Source: CAD feature listing. Evaluate the final solid. Frame: model axes, mm. Face numbers are marked on the shaded views. A direction names the side the tool comes from. Coordinates: 2 decimals unless noted, no trailing zeros. Write each loop counter-clockwise with the first axis right and the second up, starting at its lowest first coordinate (ties: lowest second). Pieces come first, ordered by that corner, then holes. Notation, with made-up numbers: (22, 18) - (37, 18) arc R24 ccw to (37, 30) - close; hole circle Ø10 at (56, 60.25). An arc over 180 degrees is marked (long way). One line per question, with ' | ' between items.
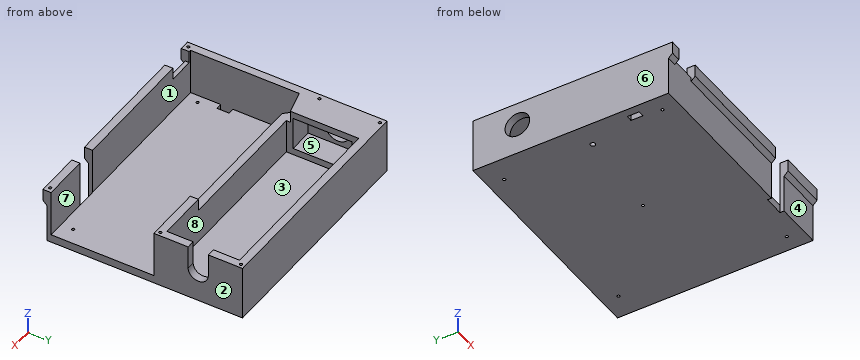
Autodesk Inventor part; units mm, degrees
ref_plane "YZ Plane" through (0, 0, 0) normal (1, 0, 0) x (0, 1, 0)
ref_plane "XZ Plane" through (0, 0, 0) normal (0, 1, 0) x (-1, 0, 0)
ref_plane "XY Plane" through (0, 0, 0) normal (0, 0, 1) x (1, 0, 0)
sketch "Skizze1" plane through (0, 0, 0) normal (0, 0, 1) x (1, 0, 0)
  line L0 (0, 0) -> (115, 0)
  line L1 (115, 0) -> (115, -97)
  line L2 (115, -97) -> (0, -97)
  line L3 (0, -97) -> (0, 0)
  dimension "d0" = 115
  dimension "d1" = 97
extrude "Extrusion1" add sketch "Skizze1" along normal blind 4
sketch "Skizze2" plane through (0, 0, 4) normal (0, 0, 1) x (1, 0, 0)
  line L0 (0, -97) -> (115, -97)
  line L1 (115, -97) -> (115, 0)
  line L2 (115, 0) -> (0, 0)
  line L3 (0, 0) -> (0, -97)
  line L4 (4, -44) -> (4, -95)
  line L5 (4, -95) -> (115, -95)
  line L6 (115, -97) -> (115, 0)
  line L7 (4, -44) -> (115, -44)
  line L8 (4, -40) -> (16, -40) construction
  line L9 (4, -40) -> (4, -36.6) construction
  line L10 (4, -4) -> (16, -4) construction
  line L11 (4, -7.4) -> (16, -7.4)
  line L12 (16, -7.4) -> (16, -4)
  line L13 (4, -36.6) -> (16, -36.6)
  line L14 (16, -36.6) -> (16, -40)
  line L15 (4, -36.6) -> (4, -7.4)
  line L16 (16, -40) -> (111, -40)
  line L17 (4, -7.4) -> (4, -4) construction
  line L18 (16, -4) -> (111, -4)
  line L19 (111, -4) -> (111, -40)
  point P0 (109.25, 0)
  point P1 (109.25, -40)
  dimension "d4" = 4
  dimension "d5" = 2
  dimension "d6" = 51
  dimension "d7" = 4
  dimension "d8" = 36
  dimension "d9" = 4
  dimension "d10" = 29.2
  dimension "d11" = 12
  dimension "d30" = 4
extrude "Extrusion2" add sketch "Skizze2" along normal blind 23 contours L3 L2 L1 L7 L4 L5 L0
sketch "Skizze4" plane through (0, 0, 4) normal (0, 0, 1) x (1, 0, 0)
  line L0 (4, -36.6) -> (16, -36.6)
  line L1 (4, -36.6) -> (16, -36.6)
  line L2 (16, -36.6) -> (16, -7.4)
  line L3 (16, -7.4) -> (4, -7.4)
  line L4 (4, -7.4) -> (4, -36.6)
  point P0 (0, 0)
  point P1 (16, -7.4)
extrude "Extrusion4" add sketch "Skizze4" along normal blind 3.3
sketch "Skizze5" plane through (4, -36.6, 27) normal (1, 0, 0) x (0, 0, -1)
  line L0 (0, 0) -> (0, 29.2)
  line L1 (0, 29.2) -> (3.3, 29.2)
  line L2 (3.3, 29.2) -> (3.3, 0)
  line L3 (3.3, 0) -> (0, 0)
  line L4 (0, 0) -> (0, 29.2)
  line L5 (19.7, 0) -> (0, 0)
  line L6 (19.7, 0) -> (19.7, 29.2)
  circle A0 centre (11.5, 14.6) radius 6.1
  line L7 (7.2229, 14.6) -> (16.7001, 14.6)
  line L8 (11.5, 24.1317) -> (11.5, 8.2548) construction
  point P0 (27, 36.6)
  dimension "d20" = 16.4
  dimension "d21" = 29.2
  dimension "d22" = 12.2
extrude "Extrusion5" cut sketch "Skizze5" against normal through all contours A0
extrude "Extrusion6" add sketch "Skizze5" along normal up to surface (12 mm away) contours L0 L1 L2 L3
sketch "Skizze6" plane through (0, 0, 27) normal (0, 0, 1) x (1, 0, 0)
  line L0 (4, -44) -> (115, -44)
  line L1 (111, -40) -> (16, -40)
  line L2 (86, -44) -> (16, -44)
  line L3 (16, -44) -> (16, -40)
  line L4 (16, -40) -> (86, -40)
  line L5 (86, -40) -> (86, -44)
  line L6 (4, -44) -> (4, -95)
  line L7 (0, -97) -> (115, -97)
  line L8 (14, -97) -> (7, -97)
  line L9 (115, -95) -> (4, -95)
  line L10 (92, -95) -> (82, -95)
  line L11 (82, -95) -> (82, -97)
  line L12 (82, -97) -> (92, -97)
  line L13 (92, -97) -> (92, -95)
  line L14 (115, -97) -> (115, -95)
  line L15 (5, -95) -> (18, -95)
  line L16 (18, -95) -> (18, -97)
  line L17 (18, -97) -> (5, -97)
  line L18 (5, -97) -> (5, -95)
  line L19 (0, 0) -> (0, -97)
  point P0 (109.25, -40)
  point P1 (86, -42)
  point P2 (86, -40)
  point P3 (82, -95)
  point P4 (5, -96)
  point P5 (18, -96)
  point P6 (5, -97)
  point P7 (18, -97)
  dimension "d27" = 70
  dimension "d41" = 10
  dimension "d42" = 23
  dimension "d65" = 13
  dimension "d66" = 5
extrude "Extrusion7" cut sketch "Skizze6" against normal blind 6 contours L3 L1 L5 L0
sketch "Skizze7" plane through (115, -97, 0) normal (1, 0, 0) x (0, 0, -1)
  arc A0 (-15.5, 80) -> (-15.5, 70) centre (-15.5, 75) ccw construction
  circle A1 centre (-15.5, 75) radius 6.1 construction
  line L0 (-15.5, 80) -> (-27, 80)
  line L1 (-27, 53) -> (-27, 97)
  line L2 (-15.5, 70) -> (-27, 70)
  arc A2 (-15.5, 70) -> (-15.5, 80) centre (-15.5, 75) ccw
  point P0 (0, 97)
  dimension "d31" = 10
extrude "Extrusion8" cut sketch "Skizze7" against normal blind 4
sketch "Skizze8" plane through (0, 0, 0) normal (0, 0, -1) x (-1, 0, 0)
  line L0 (0, -97) -> (-115, -97)
  line L1 (0, 0) -> (0, -97)
  line L2 (-115, 0) -> (0, 0)
  line L3 (-115, -97) -> (-115, 0)
  line L4 (-8, -8) -> (-8, -89) construction
  line L5 (-8, -89) -> (-107, -89) construction
  line L6 (-107, -89) -> (-107, -8) construction
  line L7 (-107, -8) -> (-8, -8) construction
  circle A0 centre (-107, -89) radius 0.7
  circle A1 centre (-8, -89) radius 0.7
  circle A2 centre (-103, -8) radius 0.7
  circle A3 centre (-12, -8) radius 0.7
  line L8 (-107, -8) -> (-8, -89) construction
  line L9 (-107, -89) -> (-8, -8) construction
  circle A4 centre (-57.5, -48.5) radius 0.7
  dimension "d34" = 8
  dimension "d35" = 1.4
  dimension "d36" = 4
  dimension "d37" = 4
extrude "Extrusion9" cut sketch "Skizze8" against normal blind 4 contours A0 | A1 | A2 | A3 | A4
extrude "Extrusion10" cut sketch "Skizze6" against normal blind 6 contours L9 L16 L7 L18
sketch "Skizze9" plane through (0, 0, 27) normal (0, 0, 1) x (1, 0, 0)
  line L0 (4, -95) -> (4, -44)
  line L1 (4, -44) -> (16, -44)
  line L2 (16, -44) -> (16, -4)
  line L3 (16, -4) -> (111, -4)
  line L4 (111, -4) -> (111, -17)
  line L5 (111, -40) -> (86, -40)
  line L6 (86, -40) -> (86, -44)
  line L7 (86, -44) -> (115, -44)
  line L8 (115, -44) -> (115, -27)
  line L9 (115, 0) -> (0, 0)
  line L10 (0, 0) -> (0, -97)
  line L11 (0, -97) -> (5, -97)
  line L12 (2.5, -2) -> (113, -2) construction
  line L13 (113, -2) -> (113, -97.1903) construction
  line L14 (113, -97.1903) -> (2.5, -97.1903) construction
  line L15 (2.5, -97.1903) -> (2.5, -2) construction
  circle A0 centre (2.5, -2) radius 0.7
  circle A1 centre (113, -2) radius 0.7
  circle A2 centre (113, -42) radius 0.7
  line L16 (113, -42) -> (2.5, -42) construction
  line L17 (4, -44) -> (16, -44) construction
  circle A3 centre (2.5, -32) radius 0.7
  line L18 (115, -27) -> (111, -27)
  line L19 (111, -27) -> (111, -40)
  line L20 (111, -17) -> (115, -17)
  line L21 (115, -17) -> (115, 0)
  line L22 (115, -97) -> (115, -95)
  line L23 (115, -95) -> (18, -95)
  line L24 (5, -97) -> (5, -95)
  line L25 (5, -95) -> (4, -95)
  line L26 (18, -95) -> (18, -97)
  line L27 (18, -97) -> (115, -97)
  dimension "d45" = 2
  dimension "d46" = 2.5
  dimension "d47" = 2
  dimension "d48" = 1.4
  dimension "d49" = 2
  dimension "d59" = 30
extrude "Extrusion11" cut sketch "Skizze9" against normal blind 4 contours A0 | A1 | A2 | A3
extrude "Extrusion12" cut sketch "Skizze6" against normal through all contours L9 L13 L7 L11
sketch "Skizze12" plane through (0, -97, 0) normal (0, -1, 0) x (1, 0, 0)
  line L0 (115, 4) -> (115, 27)
  line L1 (115, 27) -> (92, 27)
  line L2 (92, 27) -> (92, 21)
  line L3 (92, 21) -> (115, 21)
  line L4 (115, 21) -> (115, 27)
  line L5 (82, 0) -> (82, 27)
  line L6 (18, 27) -> (18, 21)
  line L7 (82, 27) -> (18, 27)
  line L8 (18, 27) -> (18, 21)
  line L9 (18, 21) -> (82, 21)
  line L10 (82, 21) -> (82, 27)
  line L11 (5, 21) -> (5, 27)
  line L12 (0, 0) -> (0, 27)
  line L13 (5, 21) -> (0, 21)
  line L14 (0, 21) -> (0, 27)
  line L15 (0, 27) -> (5, 27)
  line L16 (5, 27) -> (5, 21)
  point P0 (5, 27)
  point P1 (0, 21)
  dimension "d67" = 6
extrude "Extrusion15" add sketch "Skizze12" along normal blind 2
sketch "Skizze10" plane through (0, 0, 27) normal (0, 0, 1) x (1, 0, 0)
  line L0 (16, -44) -> (16, -4)
  line L1 (4, -44) -> (16, -44)
  line L2 (4, -95) -> (4, -44)
  line L3 (4, -44) -> (4, -41)
  line L4 (4, -41) -> (16, -38)
  point P0 (0, 0)
  dimension "d56" = 6
  dimension "d77" = 3
extrude "Extrusion13" cut sketch "Skizze10" against normal blind 6
sketch "Skizze11" plane through (0, 0, 4) normal (0, 0, 1) x (1, 0, 0)
  circle A0 centre (12, -52) radius 1.2
  line L0 (4, -44) -> (4, -95)
  line L1 (115, -44) -> (4, -44)
  point P0 (0, 0)
  dimension "d60" = 8
  dimension "d61" = 8
  dimension "d62" = 2.4
extrude "Extrusion14" cut sketch "Skizze11" against normal blind 4
sketch "Skizze13" plane through (0, 0, 27) normal (0, 0, 1) x (1, 0, 0)
  line L0 (5, -97) -> (0, -97)
  circle A0 centre (2.5, -97) radius 0.7
  circle A1 centre (2.5, -32) radius 0.7
  line L1 (0, 0) -> (0, -99)
  line L2 (115, -97) -> (92, -97)
  circle A2 centre (112.5, -97) radius 0.7
  line L3 (115, -95) -> (115, -99)
  dimension "d70" = 2.5
  dimension "d71" = 2.5
extrude "Extrusion16" cut sketch "Skizze13" against normal blind 5 contours A0 L0 | L0 A0 | A2 L2 | L2 A2
chamfer "Fasen1" distance 2 angle 45 3 edges at (2.5, -97, 21) (50, -97, 21) (103.5, -97, 21)
sketch "Skizze14" plane through (0, 0, 4) normal (0, 0, 1) x (1, 0, 0)
  line L0 (115, -44) -> (4, -44)
  line L1 (4, -74) -> (7, -74)
  line L2 (7, -74) -> (7, -80)
  line L3 (7, -80) -> (4, -80)
  line L4 (4, -80) -> (4, -44)
  line L5 (4, -95) -> (82, -95)
  point P0 (0, 0)
  point P1 (7, -44)
  point P2 (4, -74)
  dimension "d78" = 6
  dimension "d79" = 3
  dimension "d82" = 15
extrude "Extrusion17" cut sketch "Skizze14" against normal blind 10
sketch "Skizze16" plane through (0, 0, 21) normal (0, 0, 1) x (1, 0, 0)
  line L0 (86, -44) -> (4, -44)
  line L1 (4, -44) -> (4, -41)
  line L2 (4, -44) -> (4, -41)
  line L3 (4, -41) -> (9, -39.75)
  line L4 (4, -41) -> (16, -38)
  line L5 (9, -44.0784) -> (9, -39.75)
  point P0 (0, 0)
  point P1 (9, -41.9142)
  point P2 (9, -44)
  dimension "d83" = 5
extrude "Extrusion18" cut sketch "Skizze16" against normal up to surface (17 mm away)
chamfer "Fasen2" distance 4 angle 45 1 edges at (9, -44, 12.5)
properties part number "Honigschleuder_Steuerung_Netzteil"
Item 1: Ray query, line 1 along Y through (x, z) = (55, 17.75); line 2 along Y through (x, z) = (12, 1.2); line 3 along X through (y, z) = (-31.5, 19.5). Return the intervals inside material, ascending. Write a range as [from, to].
Check sheet entries:
line 1: [-97, -95], [-44, -40], [-4, 0] | line 2: [-97, -53.2], [-50.8, -8.7], [-7.3, 0] | line 3: [0, 4], [111, 115]
Item 2: Cut plane B-B on y = -60. Return loops of the section in (x, z).
Check sheet entries:
outline: (0, 0) - (115, 0) - (115, 4) - (4, 4) - (4, 27) - (0, 27) - close
Item 3: Access query for the marked faces 1, 2, 3, 4 and 5. Directions: +Z, -Z, +X, -X, +Y, -Y. A direction counts if a zero-diameter tool reaches every point of the face in a straight line with its end or side. Return the directions, or none.
Check sheet entries:
face 1: +Z, +X | face 2: +Z, -Z, +X, +Y, -Y | face 3: +Z | face 4: -Z, +X, -X, -Y | face 5: none
Item 4: Pin query (flat end, axial travel): pin 1 Ø11.5 at (x, z) = (66.5, 11.5) entering from -Y; pin 2 Ø4 at (x, z) = (89.5, 16.5) entering from -Y; pin 3 Ø2 at (x, y) = (12, -52) entering from +Z; pin 4 Ø5 at (y, z) = (-58, 7.5) entering from +X. Return the tip coordinate at first contact, or that it passes through.
Check sheet entries:
pin 1: y = -97 | pin 2: y = -44 | pin 3: through | pin 4: x = 4
Item 5: Mould query, pull axis X, two halves, no side actions, for the marked faces 6, 7 and 8. Classes: pulls with the +X half, pulls with the -X half, needs draft (parallel to the pull), parting line crosses it, or undercut.
Check sheet entries:
face 6: pulls with the -X half | face 7: needs draft | face 8: undercut
